from build123d import *

# Parameters (mm, degrees)
CROQUIS2_R              = 1.45
SALIENTE_EXTRUIR1_DEPTH = 2
CROQUIS3_W              = 16.5
CROQUIS3_H              = 9
CROQUIS3_R              = 1.45
SALIENTE_EXTRUIR2_DEPTH = 2
REDONDEO1_R             = 2
REDONDEO2_R             = 2
CROQUIS4_W              = 24
CROQUIS4_H              = 5
CORTAR_EXTRUIR1_DEPTH   = 20.535224596


with BuildPart() as part:
    # Croquis2 → Saliente-Extruir1 (new body)
    with BuildSketch(Plane(origin=(0, 0, 0), x_dir=(1, 0, 0), z_dir=(0, 1, 0))):
        Polygon((-11.25, 8.25), (11.25, 8.25), (11.25, -8.25), (-11.25, -8.25), (-13.25, -8.25), (-13.25, 8.25), align=None)
        with Locations(Location((-8, -6, 0), (0, 0, 270))):
            Circle(CROQUIS2_R, mode=Mode.SUBTRACT)
        with Locations(Location((8, -6, 0), (0, 0, 90))):
            Circle(CROQUIS2_R, mode=Mode.SUBTRACT)
    extrude(amount=SALIENTE_EXTRUIR1_DEPTH)

    # Croquis3 → Saliente-Extruir2 (add)
    with BuildSketch(Plane.ZY.offset(13.25)):
        with Locations((0, -2.5)):
            Rectangle(CROQUIS3_W, CROQUIS3_H)
        with Locations((-5, -4)):
            Circle(CROQUIS3_R, mode=Mode.SUBTRACT)
        with Locations(Location((5, -4, 0), (0, 0, 180))):
            Circle(CROQUIS3_R, mode=Mode.SUBTRACT)
    extrude(amount=SALIENTE_EXTRUIR2_DEPTH)

    # Redondeo1
    redondeo1_edges = [part.edges().sort_by_distance(p)[0] for p in [
        (-13.25, 0, 0),
    ]]
    fillet(redondeo1_edges, radius=REDONDEO1_R)

    # Redondeo2
    redondeo2_edges = [part.edges().sort_by_distance(p)[0] for p in [
        (11.25, 1, 8.25),
        (11.25, 1, -8.25),
        (-14.25, -7, -8.25),
        (-14.25, -7, 8.25),
    ]]
    fillet(redondeo2_edges, radius=REDONDEO2_R)

    # Croquis4 → Cortar-Extruir1 (cut, through all)
    with BuildSketch(Plane(origin=(0, 2, 0), x_dir=(1, 0, 0), z_dir=(0, 1, 0))):
        with Locations((-0.75, 5.75)):
            Rectangle(CROQUIS4_W, CROQUIS4_H)
    extrude(amount=-CORTAR_EXTRUIR1_DEPTH, mode=Mode.SUBTRACT)


solid = part.part
Geometry: final body of the model. Coordinates: model frame, mm. A direction names the side the tool comes from. Give positions to 0.01 mm unless a question says otherwise; leave off trailing zeros. Loops run counter-clockwise (first coordinate to the right, second up) from the corner with the lowest first, then second, coordinate; pieces in that order, holes last. Notation, with made-up numbers: (-6.5, 8.5) - (5.5, 8.5) arc R28 cw to (5.5, 31.5) - close; hole circle Ø10 at (85, -12.5). An arc over 180 degrees is marked (long way). One line per question, with ' | ' between items. Start each with the question number.
(1) Contact query for flat-ended pins moving along their axis: pin 1 (9 mm diameter, centred on x = -2.5, z = 3, fed in from -Y); pin 2 (2 mm diameter, centred on y = 1, z = -5, fed in from +X); pin 3 (0.8 mm diameter, centred on x = -3, y = 0.5, fed in from -Z). Output: stop coordinate, or through.
(2) Section query C-C on y = -4. Return loops of the section in (x, z).
(3) Ray query, line 1 (X direction, y = 1.6, z = 6); line 2 (Y direction, x = -14.2, z = -5); line 3 (Y direction, x = -4, z = 1.5). Return the intervals inside material, ascending. Write a range as from..to.
(4) Pull-direction query (Y, two-part tool) for faces 1 (the cylindrical face through (-14.24, -4.06, 6.45)), 2 (the cylindrical face through (8.88, 0.99, 7.15)), 3 (the flat face through (-2, 2, 2)); classes: released by +Y, released by -Y, zero draft, split by the parting line, or undercut.
(5) Reachability of faces 4 (the cylindrical face through (10.68, 1.01, 7.65)), 5 (the flat face through (-13.25, -4, 0)), 6 (the flat face through (-1, 1, -3.25)) from +Z, -Z, +X, -X, +Y, -Y: full face, straight path, thin tool, end or side. Return the list, or none.
(6) Section query D-D on x = 7. Return loops of the section in (y, z), then the cut area to 3 significant figures.
(7) Section query B-B on z = -5. Return loops of the section in (x, y).
(8) Section query A-A on x = -8. Return loops of the section in (y, z), then the cut area to 3 significant figures.
The answers:
1) pin 1: y = 0 | pin 2: x = -12.75 | pin 3: z = -3.25
2) outline: (-15.25, -8.25) - (-13.25, -8.25) - (-13.25, -6.45) - (-15.25, -6.45) - close; (-15.25, -3.55) - (-13.25, -3.55) - (-13.25, 3.55) - (-15.25, 3.55) - close; (-15.25, 6.45) - (-13.25, 6.45) - (-13.25, 8.25) - (-15.25, 8.25) - close
3) line 1: -15.25..-9.45, -6.55..6.55, 9.45..11.25 | line 2: -7..-5.45, -2.55..2 | line 3: 0..2
4) face 1: undercut | face 2: zero draft | face 3: released by +Y
5) face 4: +Z, +X, +Y, -Y | face 5: +Z, -Z, +X, -Y | face 6: -Z, +X, +Y, -Y
6) outline: (0, -3.25) - (2, -3.25) - (2, 4.95) - (0, 4.95) - close; (0, 7.05) - (2, 7.05) - (2, 8.25) - (0, 8.25) - close | area: 18.8 mm2
7) outline: (-15.25, -7) - (-13.25, -7) - (-13.25, -5.45) - (-15.25, -5.45) - close; (-15.25, -2.55) - (-13.25, -2.55) - (-13.25, -2) arc R2 cw to (-12.75, -0.68) - (-12.75, 2) - (-15.25, 2) - close
8) outline: (0, -3.25) - (2, -3.25) - (2, 4.55) - (0, 4.55) - close; (0, 7.45) - (2, 7.45) - (2, 8.25) - (0, 8.25) - close | area: 17.2 mm2
